Geometry: final body of the model. Coordinates: model frame, mm. A direction names the side the tool comes from. Coordinates: 2 decimals unless noted, no trailing zeros. Write each loop counter-clockwise with the first axis right and the second up, starting at its lowest first coordinate (ties: lowest second). Pieces come first, ordered by that corner, then holes.
from build123d import *

# Parameters (mm, degrees)
F0_R     = 4.3140137555
F0_R_2   = 4.7914191877
F1_DEPTH = 12.7
F2_DEPTH = 50.8
F3_R     = 4.4074532963
F4_DEPTH = 12.7
F5_R     = 4.030114566
F6_DEPTH = 25.4


# Not quite as in the source:
# - a feature names something its author has since deleted; it is built from what else it names


with BuildPart() as f1:
    # F0 (on Front) → F1 (new body)
    with BuildSketch(Plane.XZ):
        with BuildLine():
            ThreePointArc((9.5125902444, 31.9258160889), (-3.518355079, 44.9567614123), (-16.5493004024, 31.9258160889))
            Line((-16.5493004024, 31.9258160889), (-16.5493004024, -20.979821682))
            ThreePointArc((-16.5493004024, -20.979821682), (-3.518355079, -7.9488763586), (9.5125902444, -20.979821682))
            Line((9.5125902444, -20.979821682), (9.5125902444, 31.9258160889))
        make_face()
        with Locations((-3.518355079, 31.9258160889)):
            Circle(F0_R, mode=Mode.SUBTRACT)
        with BuildLine():
            ThreePointArc((9.5125902444, -20.979821682), (-3.518355079, -7.9488763586), (-16.5493004024, -20.979821682))
            ThreePointArc((-16.5493004024, -20.979821682), (-3.518355079, -34.0107670054), (9.5125902444, -20.979821682))
        make_face()
        with Locations((-3.518355079, -20.979821682)):
            Circle(F0_R_2, mode=Mode.SUBTRACT)
    extrude(amount=F1_DEPTH)

    # F0 (on Front) → F2 (join)
    with BuildSketch(Plane.XZ):
        with BuildLine():
            ThreePointArc((9.5125902444, -20.979821682), (-3.518355079, -7.9488763586), (-16.5493004024, -20.979821682))
            ThreePointArc((-16.5493004024, -20.979821682), (-3.518355079, -34.0107670054), (9.5125902444, -20.979821682))
        make_face()
        with Locations((-3.518355079, -20.979821682)):
            Circle(F0_R_2, mode=Mode.SUBTRACT)
    extrude(amount=F2_DEPTH)

    # F3 (on face) → F4 (join)
    with BuildSketch(Plane.XZ.offset(50.8)):
        with BuildLine():
            Line((-16.5491351407, 32.1166292513), (-16.5491351407, -21.0454494616))
            ThreePointArc((-16.5491351407, -21.0454494616), (-3.5857392287, -7.9490505844), (9.5124068178, -20.9106811633))
            Line((9.5124068178, -20.9106811633), (9.2310467735, 32.1166292513))
            ThreePointArc((9.2310467735, 32.1166292513), (-3.6590441836, 44.9385075287), (-16.5491351407, 32.1166292513))
        make_face()
        with Locations((-3.6590441836, 32.0482351251)):
            Circle(F3_R, mode=Mode.SUBTRACT)
        with Locations((-3.6590441836, 32.0482351251)):
            Circle(F3_R)
    extrude(amount=-F4_DEPTH)

    # F5 (on face) → F6 (cut)
    with BuildSketch(Plane.XZ.offset(50.8)):
        with Locations((-3.6590441836, 32.0482351251)):
            Circle(F5_R)
    extrude(amount=-F6_DEPTH, mode=Mode.SUBTRACT)


solid = f1.part
Item 1: Section A-A, the plane z = -6. Output: boundary loops of the cut face in (x, y).
Derived:
outline: (-16.55, -50.8) - (9.43, -50.8) - (9.43, -38.1) - (-16.55, -38.1) - close; (-16.55, -12.7) - (9.51, -12.7) - (9.51, 0) - (-16.55, 0) - close
Item 2: Set-up query: faces 1 (the flat face through (9.513, -6, 5)), 2 (the cylindrical face through (-1.82, -25.04, -33.9)), 3 (the cylindrical face through (-4.1, -6.3, 36.2)). Return all of +Z, -Z, +X, -X, +Y, -Y with unobstructed straight access to the full face (end or side cutting, diameter ignored); none if empty.
Derived:
face 1: +Z, -Z, +X, +Y, -Y
face 2: none
face 3: +Y
Item 3: Section D-D, the plane x = -15. Output: boundary loops of the cut face in (y, z).
Derived:
outline: (-50.8, -27.14) - (0, -27.14) - (0, 38.09) - (-12.7, 38.09) - (-12.7, -14.82) - (-38.1, -14.82) - (-38.1, 38.18) - (-50.8, 38.18) - close
Item 4: Pull-direction query (Y, two-part tool) for faces 4 (the flat face through (-4, -38.1, 12)), 5 (the flat face through (-4, 0, 6)), 6 (the cylindrical face through (-3.377, -44.539, 44.935)); classes: released by +Y, released by -Y, zero draft, split by the parting line, or undercut.
Derived:
face 4: undercut
face 5: released by +Y
face 6: zero draft
Item 5: Section B-B, the plane y = -9.5. Output: boundary loops of the cut face in (x, z).
Derived:
outline: (-16.55, -20.98) arc R13.03 ccw to (9.51, -20.98) - (9.51, 31.93) arc R13.03 ccw to (-16.55, 31.93) - close; hole circle Ø9.58 at (-3.52, -20.98); hole circle Ø8.63 at (-3.52, 31.93)
Item 6: Pin query (flat end, axial travel): pin 1 (7 mm diameter, centred on x = -3.52, z = 31.93, fed in from -Y); pin 2 (2 mm diameter, centred on x = 5, z = -10, fed in from +Y); pin 3 (10 mm diameter, centred on x = 3.5, y = -22, fed in from -Z); pin 4 (3 mm diameter, centred on x = 1, y = -35, fed in from +Z). Return the tip coordinate at first contact, or that it passes through.
Derived:
pin 1: passes through
pin 2: stops at y = 0
pin 3: stops at z = -33.85
pin 4: stops at z = -8.3
Item 7: Material intervals for probe 1 along Y at (x, z) = (-7.25, 19.5); probe 2 along X at (y, z) = (-34, -20); probe 3 along Z at (x, y) = (-5.25, -14), sorted ascending.
Derived:
probe 1: y = -50.8 to -38.1, -12.7 to 0
probe 2: x = -16.51 to -8.21, 1.17 to 9.48
probe 3: z = -33.9 to -25.45, -16.51 to -8.06
Item 8: Section C-C, the plane x = -1.75. Output: boundary loops of the cut face in (y, z).
Derived:
outline: (-50.8, -33.89) - (0, -33.89) - (0, -25.43) - (-50.8, -25.43) - close; (-50.8, -16.53) - (0, -16.53) - (0, 27.99) - (-12.7, 27.99) - (-12.7, -8.07) - (-38.1, -8.07) - (-38.1, 28.5) - (-50.8, 28.5) - close; (-50.8, 35.6) - (-38.1, 35.6) - (-38.1, 44.8) - (-50.8, 44.8) - close; (-12.7, 35.86) - (0, 35.86) - (0, 44.84) - (-12.7, 44.84) - close
